Geometry: final body of the model. Coordinates: model frame, mm. Face numbers are marked on the shaded views. A direction names the side the tool comes from. Coordinates: 2 decimals unless noted, no trailing zeros. Order: outer loops, then holes, each group sorted by start corner. A loop starts at its lowest first (then second) coordinate and runs counter-clockwise, first axis right, second up. Notation, with made-up numbers: M -24.75,47 L 22.25,47 A18 ccw 22.25,57 Z; hole C 38.5,-28 d1. An arc over 180 degrees is marked long. Use CSV: the item, a comma, the result in double quotes. Start each with the question number.
Q1. Section query B-B, the plane z = 9.75. Output: boundary loops of the cut face in (x, y).
Q2. First-contact query: P1, Ø4, axis at x = -9.5, z = 11, coming from the -Y side; P2, Ø1, axis at y = 12.5, z = 11, coming from the +X side; P3, Ø8, axis at x = 69, z = 2, coming from the -Y side. Flat tips, straight axial feed; report the tip coordinate or a pass-through.
Q3. Section query D-D, the plane y = 10. Output: boundary loops of the cut face in (x, z).
Q4. Access query for the marked faces 4 and 5. Directions: +Z, -Z, +X, -X, +Y, -Y. A direction counts if a zero-diameter tool reaches every point of the face in a straight line with its end or side. Return the directions, or none.
Q5. Section query A-A, the plane x = 34.5. Output: boundary loops of the cut face in (y, z), and give its area (3 significant figures).
Q6. Ray query, probe 1 along X at (y, z) = (0, 11.75); probe 2 along X at (y, z) = (-46.5, 5.5); probe 3 along Y at (x, z) = (-73, 5). Return the intervals inside material, ascending.
Q7. Mould query, pull axis X, two halves, no side actions, for the marked faces 1, 2 and 3. Classes: +X half, -X half, draft (parallel to the pull), parting line (faces both ways), or undercut.
Q8. Section query C-C, the plane y = 40. Output: boundary loops of the cut face in (x, z).
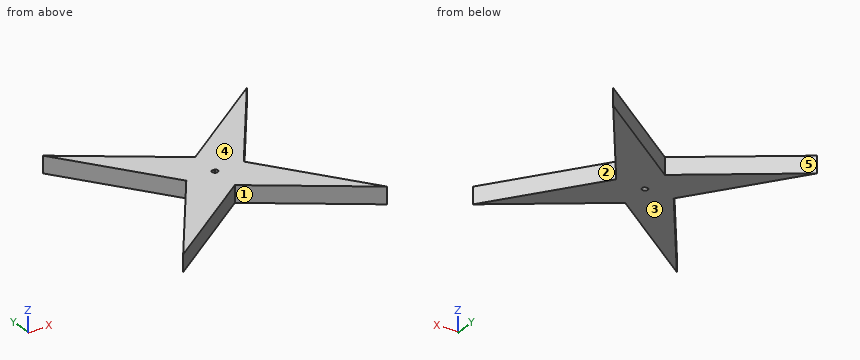
Autodesk Inventor part; units mm, degrees
ref_plane "YZ Plane" through (0, 0, 0) normal (1, 0, 0) x (0, 1, 0)
ref_plane "XZ Plane" through (0, 0, 0) normal (0, 1, 0) x (-1, 0, 0)
ref_plane "XY Plane" through (0, 0, 0) normal (0, 0, 1) x (1, 0, 0)
sketch "Sketch1" plane through (0, 0, 0) normal (0, 0, 1) x (1, 0, 0)
  arc A0 (-1.473, 2.02) -> (1.473, 2.02) centre (0, 0) ccw
  line L0 (0, 2.5) -> (0, 2.02)
  line L1 (0, 2.02) -> (1.473, 2.02)
  line L2 (0, 2.02) -> (-1.473, 2.02)
  line L3 (0, 0) -> (125, 0) construction
  line L4 (88.3883, 88.3883) -> (0.0691, 24.9999)
  line L5 (-88.2502, 88.3883) -> (0.0691, 24.9999)
  line L6 (0.0691, 24.9999) -> (-88.2502, 88.3883)
  line L7 (88.3883, 88.3883) -> (0.0691, 24.9999)
  line L8 (25, 0) -> (88.3883, 88.3883)
  line L9 (-24.9987, 0.2597) -> (-88.2502, 88.3883)
  line L10 (0, 0) -> (7.0052, 0)
  line L11 (88.3883, -88.3883) -> (0.0691, -24.9999)
  line L12 (-88.2502, -88.3883) -> (0.0691, -24.9999)
  line L13 (25, 0) -> (88.3883, -88.3883)
  line L14 (-24.9987, -0.2597) -> (-88.2502, -88.3883)
  line L15 (0.0691, -24.9999) -> (-88.2502, -88.3883)
  line L16 (-88.2502, -88.3883) -> (-24.9987, -0.2597)
  line L17 (88.3883, -88.3883) -> (0.0691, -24.9999)
  line L18 (88.3883, -88.3883) -> (25, 0)
  line L19 (88.3883, -88.3883) -> (0.0691, -24.9999)
  line L20 (0.0691, -24.9999) -> (-88.2502, -88.3883)
  line L21 (-88.2502, -88.3883) -> (-24.9987, -0.2597)
  line L22 (-24.9987, -0.2597) -> (-24.8122, 0)
  line L23 (-24.8122, 0) -> (-24.9987, 0.2597)
  dimension "d0" = 5
  dimension "d1" = 0.48
  dimension "d3" = 125
extrude "Extrusion1" add sketch "Sketch1" along normal blind 14.5
sketch "Sketch2" plane through (0, 0, 14.5) normal (0, 0, 1) x (1, 0, 0)
  line L0 (0.0691, 24.9999) -> (-88.2502, 88.3883)
  line L1 (0.0691, 24.9999) -> (-88.2502, 88.3883)
  line L2 (88.3883, 88.3883) -> (0.0691, 24.9999)
  line L3 (-88.2502, 88.3883) -> (88.3883, 88.3883)
  line L4 (88.3883, 88.3883) -> (0.0691, 24.9999)
  point P0 (0, 0)
properties part number "Dispensing Gear"
Responses:
1,outline,"M -88.25,-88.39 L 0.07,-25 L 88.39,-88.39 L 25,0 L 88.39,88.39 L 0.07,25 L -88.25,88.39 L -25,0.26 L -24.81,0 L -25,-0.26 Z; hole M -1.47,2.02 A2.5 ccw long 1.47,2.02 Z"
2,P1,"stops at y = -33.3"
2,P2,"stops at x = 34.32"
2,P3,"stops at y = -77.34"
3,outline,"M -31.99,0 L 32.17,0 L 32.17,14.5 L -31.99,14.5 Z"
4,face 4,"+Z, +X, -X, +Y, -Y"
4,face 5,"+Z, -Z, +Y"
5,outline,"M -49.71,0 L -13.25,0 L -13.25,14.5 L -49.71,14.5 Z; M 13.25,0 L 49.71,0 L 49.71,14.5 L 13.25,14.5 Z"
5,area,"1,060 mm²"
6,probe 1,"x = -24.81 to -2.5, 2.5 to 25"
6,probe 2,"x = -58.19 to -29.89, 30.03 to 58.35"
6,probe 3,"y = -77.44 to -67.14, 67.14 to 77.44"
7,face 1,"undercut"
7,face 2,"+X half"
7,face 3,"draft"
8,outline,"M -53.52,0 L -20.83,0 L -20.83,14.5 L -53.52,14.5 Z; M 20.97,0 L 53.69,0 L 53.69,14.5 L 20.97,14.5 Z"
